Here's how the part is built. I have some questions about the finished solid (model axes, mm). A direction names the side the tool comes from. Give positions to 0.01 mm unless a question says otherwise; leave off trailing zeros. Loops run counter-clockwise (first coordinate to the right, second up) from the corner with the lowest first, then second, coordinate; pieces in that order, holes last.
Q1. Thinking about a two-plate mould opening in X: for faces 3 (the face through (-28.059, -82.556, 1.479)), 4 (the face through (-25, -6, 0)), 5 (the face through (28.51, 28.25, 1.48)), which applies, pulls with the +X half, pulls with the -X half, needs draft (parallel to the pull), parting line crosses it, or undercut?
Q2. I need wall thicknesses on probe 1 along X at (y, z) = (58, 0.2); probe 2 along X at (y, z) = (77.5, 0.8); probe 3 along X at (y, z) = (13, 2.15). Which ranges of each line are inside material? Lowest first, please.
Q3. Suppose I cut it at D-D (x = -48). List the corners of the cut face in (y, z) for me.
Q4. For faces 1 (the face through (-25, -6, 3)), 2 (the face through (-28.604, -28.231, 1.479)), which set-ups out of +Z, -Z, +X, -X, +Y, -Y let a thin tool reach every point of the face, with its end or its side?
Q5. Suppose I cut it at C-C (y = -69). List the corners of the cut face in (x, z) for me.
Q6. I'm going to push flat-ended pins straight in: P1, Ø0.9, axis at x = 68, z = 2, coming from the -Y side; P2, Ø0.9, axis at y = 59, z = 1.5, coming from the -X side; P3, Ø1.5, axis at y = 83.5, z = 2, coming from the -X side; P4, Ø3.5, axis at x = -27.14, y = -80.78, coming from the -Z side. Where does each tip first touch, or does it pass through?
Q7. Suppose I cut it at A-A (y = 0). List the corners of the cut face in (x, z) for me, and give its area (3 significant figures).
Q8. Suppose I cut it at B-B (x = 0). List the corners of the cut face in (y, z) for me.
```python
from build123d import *

# Parameters (mm, degrees)
CROQUIS1_R              = 25
SALIENTE_EXTRUIR1_DEPTH = 3
CROQUIS2_W              = 12.95
CROQUIS2_H              = 12.95
SALIENTE_EXTRUIR2_DEPTH = 3
CROQUIS3_R              = 2
CORTAR_EXTRUIR1_DEPTH   = 124.455998815


with BuildPart() as part:
    # Croquis1 → Saliente-Extruir1 (new body)
    with BuildSketch(Plane.XY):
        with BuildLine():
            Line((-15.070986718, 74.306476298), (-15.070986718, 37.256476298))
            ThreePointArc((-15.070986718, 37.256476298), (-28.445175059, 28.391049341), (-37.285113206, 15))
            Line((-37.285113206, 15), (-74.335113206, 15))
            Line((-74.335113206, 15), (-74.335113206, 20.59))
            Line((-74.335113206, 20.59), (-87.285113206, 20.59))
            Line((-87.285113206, 20.59), (-87.285113206, -20.59))
            Line((-87.285113206, -20.59), (-74.335113206, -20.59))
            Line((-74.335113206, -20.59), (-74.335113206, -15))
            Line((-74.335113206, -15), (-37.285113206, -15))
            ThreePointArc((-37.285113206, -15), (-28.445175059, -28.391049341), (-15.070986718, -37.256476298))
            Line((-15.070986718, -37.256476298), (-15.070986718, -74.306476298))
            Line((-15.070986718, -74.306476298), (-20.660986718, -74.306476298))
            Line((-20.660986718, -74.306476298), (-20.660986718, -87.256476298))
            Line((-20.660986718, -87.256476298), (20.519013282, -87.256476298))
            Line((20.519013282, -87.256476298), (20.519013282, -74.306476298))
            Line((20.519013282, -74.306476298), (14.929013282, -74.306476298))
            Line((14.929013282, -74.306476298), (14.929013282, -37.256476298))
            ThreePointArc((14.929013282, -37.256476298), (28.353570497, -28.407666286), (37.22795272, -15))
            Line((37.22795272, -15), (59.27795272, -15))
            Line((59.27795272, -15), (59.27795272, -20.59))
            Line((59.27795272, -20.59), (72.22795272, -20.59))
            Line((72.22795272, -20.59), (72.22795272, 20.59))
            Line((72.22795272, 20.59), (59.27795272, 20.59))
            Line((59.27795272, 20.59), (59.27795272, 15))
            Line((59.27795272, 15), (37.22795272, 15))
            ThreePointArc((37.22795272, 15), (28.353570497, 28.407666286), (14.929013282, 37.256476298))
            Line((14.929013282, 37.256476298), (14.929013282, 74.306476298))
            Line((14.929013282, 74.306476298), (20.519013282, 74.306476298))
            Line((20.519013282, 74.306476298), (20.519013282, 87.256476298))
            Line((20.519013282, 87.256476298), (-20.660986718, 87.256476298))
            Line((-20.660986718, 87.256476298), (-20.660986718, 74.306476298))
            Line((-20.660986718, 74.306476298), (-15.070986718, 74.306476298))
        make_face()
        Circle(CROQUIS1_R, mode=Mode.SUBTRACT)
    extrude(amount=SALIENTE_EXTRUIR1_DEPTH)

    # Croquis2 → Saliente-Extruir2 (add)
    with BuildSketch(Plane(origin=(0, 0, 0), x_dir=(-1, 0, 0), z_dir=(0, 0, -1))):
        with Locations((-26.994013282, 80.781476298)):
            Rectangle(CROQUIS2_W, CROQUIS2_H)
        with Locations((27.135986718, 80.781476298)):
            Rectangle(CROQUIS2_W, CROQUIS2_H)
        with Locations((-26.994013282, -80.781476298)):
            Rectangle(CROQUIS2_W, CROQUIS2_H)
        with Locations((27.135986718, -80.781476298)):
            Rectangle(CROQUIS2_W, CROQUIS2_H)
        with Locations((80.810113206, 27.065)):
            Rectangle(CROQUIS2_W, CROQUIS2_H)
        with Locations((80.810113206, -27.065)):
            Rectangle(CROQUIS2_W, CROQUIS2_H)
    extrude(amount=-SALIENTE_EXTRUIR2_DEPTH)

    # Croquis3 → Cortar-Extruir1 (cut, through all)
    with BuildSketch(Plane(origin=(0, 0, 0), x_dir=(-1, 0, 0), z_dir=(0, 0, -1))):
        with Locations((-26.994013282, 80.781476298)):
            Circle(CROQUIS3_R)
        with Locations((27.135986718, 80.781476298)):
            Circle(CROQUIS3_R)
        with Locations((27.135986718, -80.781476298)):
            Circle(CROQUIS3_R)
        with Locations((-26.994013282, -80.781476298)):
            Circle(CROQUIS3_R)
        with Locations((80.810113206, -27.065)):
            Circle(CROQUIS3_R)
        with Locations((80.810113206, 27.065)):
            Circle(CROQUIS3_R)
    extrude(amount=-CORTAR_EXTRUIR1_DEPTH, mode=Mode.SUBTRACT)


solid = part.part
```
Solutions:
1. face 3: undercut
1. face 4: needs draft
1. face 5: undercut
2. probe 1: x = -15.07 to 14.93
2. probe 2: x = -33.61 to 33.47
2. probe 3: x = -87.29 to -21.35, 21.35 to 72.23
3. outline: (-15, 0) - (15, 0) - (15, 3) - (-15, 3) - close
4. face 1: +Z, +X, -X, +Y, -Y
4. face 2: +Z, -Z
5. outline: (-15.07, 0) - (14.93, 0) - (14.93, 3) - (-15.07, 3) - close
6. P1: stops at y = -20.59
6. P2: stops at x = -15.07
6. P3: stops at x = -33.61
6. P4: passes through
7. outline: (-87.29, 0) - (-25, 0) - (-25, 3) - (-87.29, 3) - close; (25, 0) - (72.23, 0) - (72.23, 3) - (25, 3) - close
7. area: 329 mm2
8. outline: (-87.26, 0) - (-25, 0) - (-25, 3) - (-87.26, 3) - close; (25, 0) - (87.26, 0) - (87.26, 3) - (25, 3) - close
